from build123d import *

# Parameters (mm, degrees)
SKETCH1_W           = 106
SKETCH1_H           = 127
SKETCH1_R           = 1.64973
SKETCH1_R_2         = 1.746
BOSS_EXTRUDE1_DEPTH = 12.7


with BuildPart() as part:
    # Sketch1 → Boss-Extrude1 (new body)
    with BuildSketch(Plane.XY):
        with Locations((53, 12.7)):
            Rectangle(SKETCH1_W, SKETCH1_H)
        with Locations((82.698486542, 55.898482492)):
            Circle(SKETCH1_R, mode=Mode.SUBTRACT)
        with Locations((95.00000245, 26.19999595)):
            Circle(SKETCH1_R_2, mode=Mode.SUBTRACT)
        with Locations((82.698486542, -3.498490592)):
            Circle(SKETCH1_R, mode=Mode.SUBTRACT)
        with Locations((23.301513458, -3.498490592)):
            Circle(SKETCH1_R, mode=Mode.SUBTRACT)
        with Locations((10.99999755, 26.1999984)):
            Circle(SKETCH1_R_2, mode=Mode.SUBTRACT)
        with Locations((23.301513458, 55.898482492)):
            Circle(SKETCH1_R, mode=Mode.SUBTRACT)
        with Locations((53, 68.1999984)):
            Circle(SKETCH1_R, mode=Mode.SUBTRACT)
        with BuildLine():
            Line((34.25, -6.275954242), (34.25, -25.4))
            Line((34.25, -25.4), (71.75, -25.4))
            Line((71.75, -25.4), (71.75, -6.275954242))
            ThreePointArc((71.75, -6.275954242), (53, 63.6999984), (34.25, -6.275954242))
        make_face(mode=Mode.SUBTRACT)
    extrude(amount=BOSS_EXTRUDE1_DEPTH)


solid = part.part
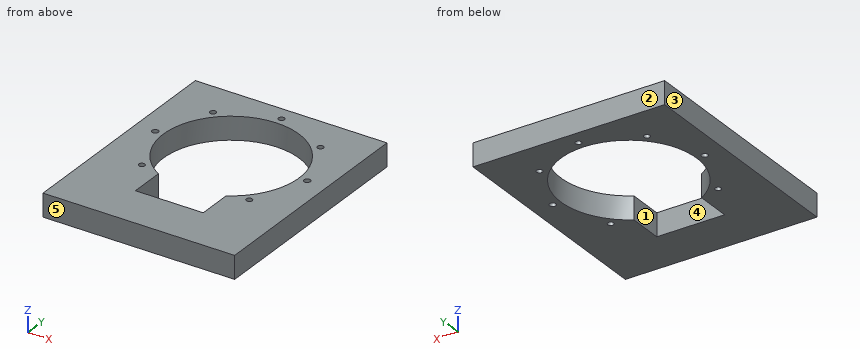
For this review, take the finished solid that the model builds, in its own axes (mm). Face numbers are marked on the shaded views. A direction names the side the tool comes from. Coordinates: 2 decimals unless noted, no trailing zeros. Loops run counter-clockwise (first coordinate to the right, second up) from the corner with the lowest first, then second, coordinate; pieces in that order, holes last. Notation, with made-up numbers: (19, 46.25) - (69, 46.25) arc R18 ccw to (69, 54.25) - close; hole circle Ø5 at (-7, -22). An arc over 180 degrees is marked (long way). Use a Markdown table: item, result. Add a question column.
Item 1: We need section C-C (z = 4). Give the number of separate pieces and of enclosed holes in the cut face, and give its area (3 significant figures).
Item 2: We need section B-B (y = -11). Give the boundary of the cut face in (x, z).
Item 3: For line 1 (Y direction, x = 53, z = 8.5); line 2 (X direction, y = -22, z = 8.75); line 3 (Y direction, x = 52, z = 7.5), list the stretches that pass through material, from the lowest coordinate up.
Item 4: We need section A-A (x = 53). Give the boundary of the cut face in (y, z).
Item 5: Tool access review of the marked faces 1 and 2: name each direction out of +Z, -Z, +X, -X, +Y, -Y from which nothing blocks a thin tool from reaching the whole face with its end or side.
Item 6: Mouldability with a two-part tool opening along Y and no side actions: class the marked faces 3, 4 and 5 as pulls with the +Y half, pulls with the -Y half, needs draft (parallel to the pull), parting line crosses it, or undercut.
Results list:
| question | item | result |
|---|---|---|
| 1 | separate pieces | 1 |
| 1 | enclosed holes | 8 |
| 1 | area | 8,390 mm^2 |
| 2 | outline | (0, 0) - (34.25, 0) - (34.25, 12.7) - (0, 12.7) - close; (71.75, 0) - (106, 0) - (106, 12.7) - (71.75, 12.7) - close |
| 3 | line 1 | y = -50.8 to -25.4, 63.7 to 66.55, 69.85 to 76.2 |
| 3 | line 2 | x = 0 to 34.25, 71.75 to 106 |
| 3 | line 3 | y = -50.8 to -25.4, 63.69 to 66.89, 69.51 to 76.2 |
| 4 | outline | (-50.8, 0) - (-25.4, 0) - (-25.4, 12.7) - (-50.8, 12.7) - close; (63.7, 0) - (66.55, 0) - (66.55, 12.7) - (63.7, 12.7) - close; (69.85, 0) - (76.2, 0) - (76.2, 12.7) - (69.85, 12.7) - close |
| 5 | face 1 | +Z, -Z |
| 5 | face 2 | +Z, -Z, +X, -X, +Y |
| 6 | face 3 | needs draft |
| 6 | face 4 | undercut |
| 6 | face 5 | pulls with the -Y half |
